Here's how the part is built. I have some questions about the finished solid (model axes, mm). Round coordinates to 2 decimals unless told otherwise and drop trailing zeros. Loops run counter-clockwise (first coordinate to the right, second up) from the corner with the lowest first, then second, coordinate; pieces in that order, holes last. Notation, with made-up numbers: M 89.5,-29.75 L 113.5,-29.75 A18 cw 113.5,-22.75 Z; hole C 2,-38.5 d3. An arc over 180 degrees is marked long. Write each question's results on one line, items separated by ' | '. Start each with the question number.
```python
from build123d import *

# Parameters (mm, degrees)
F1_DEPTH = 1


with BuildPart() as f1:
    # F0 (on Top) → F1 (new body)
    with BuildSketch(Plane.XY):
        with BuildLine():
            ThreePointArc((-27.3388900485, -0.9977917653), (-27.2922865727, -0.6055926478), (-27.2767198383, -0.2109412719))
            ThreePointArc((-27.2767198383, -0.2109412719), (-27.3156011331, 0.4120452206), (-27.4316415742, 1.0253628716))
            ThreePointArc((-27.4316415742, 1.0253628716), (-27.8797003635, 2.1720812966), (-28.5938661896, 3.1749207641))
            ThreePointArc((-28.5938661896, 3.1749207641), (-37.2855795833, -0.5574762051), (-28.1619703008, -3.0547592313))
            ThreePointArc((-28.1619703008, -3.0547592313), (-27.6353110241, -2.0723395713), (-27.3388900485, -0.9977917653))
        make_face()
        with BuildLine():
            ThreePointArc((-29.0279696038, -1.4164111001), (-35.823533245, -0.271588351), (-29.0587042579, 1.0427149257))
            Line((-29.0587042579, 1.0427149257), (-27.4248942733, -0.2084955195))
            Line((-27.4248942733, -0.2084955195), (-29.0279696038, -1.4164111001))
        make_face(mode=Mode.SUBTRACT)
        with BuildLine():
            ThreePointArc((-27.4316415742, 1.0253628716), (-27.3156011331, 0.4120452206), (-27.2767198383, -0.2109412719))
            ThreePointArc((-27.2767198383, -0.2109412719), (-27.2922865727, -0.6055926478), (-27.3388900485, -0.9977917653))
            Line((-27.3388900485, -0.9977917653), (-26.0078907013, -0.9977917653))
            Line((-26.0078907013, -0.9977917653), (-1.021916396, -0.9977917653))
            Line((-1.021916396, -0.9977917653), (-1.021916396, 1.0253628716))
            Line((-1.021916396, 1.0253628716), (-26.0030180216, 1.0253628716))
            Line((-26.0030180216, 1.0253628716), (-27.4316415742, 1.0253628716))
        make_face()
        with BuildLine():
            ThreePointArc((-28.5938661896, 3.1749207641), (-27.8797003635, 2.1720812966), (-27.4316415742, 1.0253628716))
            Line((-27.4316415742, 1.0253628716), (-26.0030180216, 1.0253628716))
            Line((-26.0030180216, 1.0253628716), (-28.5938661896, 3.1749207641))
        make_face()
        with BuildLine():
            Line((-26.0078907013, -0.9977917653), (-27.3388900485, -0.9977917653))
            ThreePointArc((-27.3388900485, -0.9977917653), (-27.6353110241, -2.0723395713), (-28.1619703008, -3.0547592313))
            Line((-28.1619703008, -3.0547592313), (-26.0078907013, -0.9977917653))
        make_face()
        Polygon((0.9874751559, 1.0253628716), (-1.021916396, 1.0253628716), (-1.021916396, -0.9977917653), (1.015001093, -1.0115547339), align=None)
        with BuildLine():
            Line((-1.021916396, 25.9902365506), (-1.021916396, 1.0253628716))
            Line((-1.021916396, 1.0253628716), (0.9874751559, 1.0253628716))
            Line((0.9874751559, 1.0253628716), (0.9874751559, 25.9992666543))
            Line((0.9874751559, 25.9992666543), (3.1274161369, 28.2286134091))
            ThreePointArc((3.1274161369, 28.2286134091), (-0.2110990703, 27.1480978017), (-3.4350626667, 28.5334701326))
            Line((-3.4350626667, 28.5334701326), (-1.021916396, 25.9902365506))
        make_face()
        with BuildLine():
            Line((1.015001093, -1.0115547339), (-1.021916396, -0.9977917653))
            Line((-1.021916396, -0.9977917653), (-1.021916396, -25.9947646409))
            Line((-1.021916396, -25.9947646409), (-3.6052718224, -28.6383550821))
            ThreePointArc((-3.6052718224, -28.6383550821), (-0.1318413861, -27.131580678), (3.4036372353, -28.4863791938))
            Line((3.4036372353, -28.4863791938), (1.015001093, -25.9817112237))
            Line((1.015001093, -25.9817112237), (1.015001093, -1.0115547339))
        make_face()
        with BuildLine():
            Line((25.9883347899, 1.0253628716), (0.9874751559, 1.0253628716))
            Line((0.9874751559, 1.0253628716), (1.015001093, -1.0115547339))
            Line((1.015001093, -1.0115547339), (25.9923934937, -1.0115547339))
            Line((25.9923934937, -1.0115547339), (28.6975805016, -3.5872808494))
            ThreePointArc((28.6975805016, -3.5872808494), (27.369536281, -0.1344353197), (28.8009183125, 3.2768678307))
            Line((28.8009183125, 3.2768678307), (25.9883347899, 1.0253628716))
        make_face()
        with BuildLine():
            ThreePointArc((5.0084020941, 32.1307584701), (-1.9347123757, 36.7196739343), (-3.4350626667, 28.5334701326))
            ThreePointArc((-3.4350626667, 28.5334701326), (-0.2110990703, 27.1480978017), (3.1274161369, 28.2286134091))
            ThreePointArc((3.1274161369, 28.2286134091), (4.5136154985, 29.9648380971), (5.0084020941, 32.1307584701))
        make_face()
        with BuildLine():
            ThreePointArc((-1.2298567505, 28.8454476519), (-2.0094686913, 35.0154222768), (3.5018862947, 32.1342163019))
            ThreePointArc((3.5018862947, 32.1342163019), (2.8835722571, 30.1450564857), (1.2465469638, 28.8569504291))
            Line((1.2465469638, 28.8569504291), (0, 27.2457357496))
            Line((0, 27.2457357496), (-1.2298567505, 28.8454476519))
        make_face(mode=Mode.SUBTRACT)
        with BuildLine():
            ThreePointArc((3.4036372353, -28.4863791938), (-0.1318413861, -27.131580678), (-3.6052718224, -28.6383550821))
            ThreePointArc((-3.6052718224, -28.6383550821), (-1.9131855373, -36.7768054017), (4.9850663184, -32.1387399713))
            ThreePointArc((4.9850663184, -32.1387399713), (4.6761248214, -30.4069429432), (3.7874147234, -28.8887992883))
            Line((3.7874147234, -28.8887992883), (3.4036372353, -28.4863791938))
        make_face()
        with BuildLine():
            ThreePointArc((1.2534396715, -28.8638722912), (2.8530229788, -30.1549993601), (3.4550732676, -32.1205047187))
            ThreePointArc((3.4550732676, -32.1205047187), (-2.102698937, -34.9700851409), (-1.1725544757, -28.7940207192))
            Line((-1.1725544757, -28.7940207192), (0, -27.6099070907))
            Line((0, -27.6099070907), (1.2534396715, -28.8638722912))
        make_face(mode=Mode.SUBTRACT)
        with BuildLine():
            ThreePointArc((37.2871905838, -0.209084826), (34.2123813861, 4.378089767), (28.8009183125, 3.2768678307))
            ThreePointArc((28.8009183125, 3.2768678307), (27.369536281, -0.1344353197), (28.6975805016, -3.5872808494))
            ThreePointArc((28.6975805016, -3.5872808494), (34.1431171019, -4.8241040496), (37.2871905838, -0.209084826))
        make_face()
        with BuildLine():
            ThreePointArc((29.0519181081, 1.062034124), (32.9656955311, 3.2370827906), (35.8250662459, -0.2085651216))
            ThreePointArc((35.8250662459, -0.2085651216), (32.947537117, -3.6575699539), (29.0387142098, -1.4446732776))
            Line((29.0387142098, -1.4446732776), (27.4487081915, -0.1906345278))
            Line((27.4487081915, -0.1906345278), (29.0519181081, 1.062034124))
        make_face(mode=Mode.SUBTRACT)
        with BuildLine():
            ThreePointArc((3.7874147234, -28.8887992883), (3.6011154409, -28.6822587182), (3.4036372353, -28.4863791938))
            Line((3.4036372353, -28.4863791938), (3.7874147234, -28.8887992883))
        make_face()
    extrude(amount=F1_DEPTH)


solid = f1.part
```
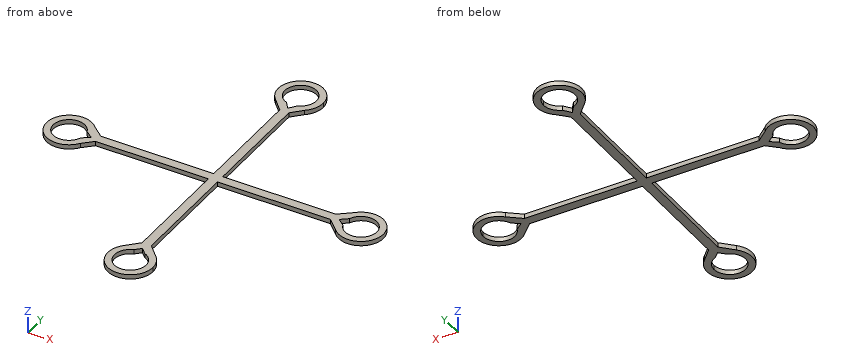
1. I want a section at B-B on z = 0.75. Count the separate pieces of the cut face and the enclosed holes in it, plus the area to 3 significant figures.
2. I want a section at A-A on x = 31.5. List the corners of the cut face in (y, z) for me.
3. I want a section at D-D on x = 8.5. List the corners of the cut face in (y, z) for me.
4. I want a section at C-C on y = 24. List the corners of the cut face in (x, z) for me.
5. For pin 1 (0.5 mm diameter, centred on x = 10.5, z = 0.5, fed in from +Y); pin 2 (0.5 mm diameter, centred on y = 13.5, z = 0.5, fed in from +X); pin 3 (4 mm diameter, centred on x = -0.01, y = 32.13, fed in from +Z), each with a flat end and sliding along its axis, tell me the tip position at first contact or that it passes through.
6. I need wall thicknesses on line 1 along Y through (x, z) = (2, 0.5); line 2 along Y through (x, z) = (-18.5, 0.15); line 3 along Y through (x, z) = (-32, 0.6). Which ranges of each line are inside material? Lowest first, please.
Outcome:
1) separate pieces: 1 | enclosed holes: 4 | area: 380 mm2
2) outline: M -5.1,0 L -3.62,0 L -3.62,1 L -5.1,1 Z; M 3.2,0 L 4.68,0 L 4.68,1 L 3.2,1 Z
3) outline: M -1.01,0 L 1.03,0 L 1.03,1 L -1.01,1 Z
4) outline: M -1.02,0 L 0.99,0 L 0.99,1 L -1.02,1 Z
5) pin 1: y = 1.03 | pin 2: x = 0.99 | pin 3: through
6) line 1: -36.72 to -34.97, -29.28 to -27.01, -1.01 to 1.03, 27.05 to 29.26, 35.01 to 36.71 | line 2: -1 to 1.03 | line 3: -5.21 to -3.71, 3.26 to 4.79
